```python
from build123d import *

# Parameters (mm, degrees)
BOSS_EXTRUDE1_DEPTH     = 6
CUT_EXTRUDE1_START      = 3
SKETCH2_R               = 8.25
CUT_EXTRUDE1_DEPTH      = 3
CUT_EXTRUDE2_REACH      = 14
SKETCH3_R               = 1.75
SKETCH4_R               = 3
CUT_EXTRUDE3_DEPTH      = 1
CUT_EXTRUDE3_DEPTH_BACK = 3


with BuildPart() as part:
    # Sketch1 → Boss-Extrude1 (new body, symmetric)
    with BuildSketch(Plane(origin=(0, 0, 0), x_dir=(1, 0, 0), z_dir=(0, 1, 0))):
        with BuildLine():
            Line((-6.25, 0), (-18.75, 0))
            Line((-18.75, 0), (-18.75, 12))
            Line((-18.75, 12), (18.75, 12))
            Line((18.75, 12), (18.75, 0))
            Line((18.75, 0), (6.25, 0))
            ThreePointArc((6.25, 0), (0, 6.25), (-6.25, 0))
        make_face()
    extrude(amount=BOSS_EXTRUDE1_DEPTH, both=True)

    # Sketch2 → Cut-Extrude1 (cut)
    with BuildSketch(Plane(origin=(0, 0, 0), x_dir=(1, 0, 0), z_dir=(0, 1, 0)).offset(CUT_EXTRUDE1_START)):
        Circle(SKETCH2_R)
    cut_extrude1 = extrude(amount=CUT_EXTRUDE1_DEPTH, mode=Mode.SUBTRACT)

    # Mirror1: Cut-Extrude1 across plane
    add(cut_extrude1.mirror(Plane.ZX), mode=Mode.SUBTRACT)

    # Sketch3 → Cut-Extrude2 (cut, up to next)
    with BuildSketch(Plane.XY, mode=Mode.PRIVATE) as cut_extrude2_sk1:
        with Locations((-11.25, 0)):
            Circle(SKETCH3_R)
    cut_extrude2_tool1 = extrude(cut_extrude2_sk1.sketch, amount=-CUT_EXTRUDE2_REACH, mode=Mode.PRIVATE) & part.part
    add(cut_extrude2_tool1.solids().sort_by_distance((-11.25, 0, 0))[0], mode=Mode.SUBTRACT)
    # Sketch3 → Cut-Extrude2 (cut, up to next)
    with BuildSketch(Plane.XY, mode=Mode.PRIVATE) as cut_extrude2_sk2:
        with Locations((11.25, 0)):
            Circle(SKETCH3_R)
    cut_extrude2_tool2 = extrude(cut_extrude2_sk2.sketch, amount=-CUT_EXTRUDE2_REACH, mode=Mode.PRIVATE) & part.part
    add(cut_extrude2_tool2.solids().sort_by_distance((11.25, 0, 0))[0], mode=Mode.SUBTRACT)

    # Sketch4 → Cut-Extrude3 (cut, two sides)
    with BuildSketch(Plane(origin=(0, 0, -12), x_dir=(-1, 0, 0), z_dir=(0, 0, -1))) as cut_extrude3_sk:
        with Locations((11.25, 0)):
            Circle(SKETCH4_R)
        with Locations((-11.25, 0)):
            Circle(SKETCH4_R)
    extrude(amount=CUT_EXTRUDE3_DEPTH, mode=Mode.SUBTRACT)
    extrude(cut_extrude3_sk.sketch, amount=-CUT_EXTRUDE3_DEPTH_BACK, mode=Mode.SUBTRACT)


solid = part.part
```
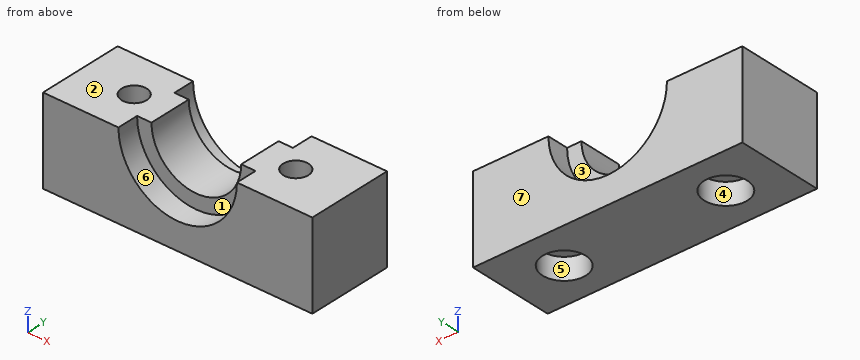
CAD build for the part. Positions are in the model's coordinates, mm. Face numbers are marked on the shaded views. A direction names the side the tool comes from. Round coordinates to 2 decimals unless told otherwise and drop trailing zeros. Loops run counter-clockwise (first coordinate to the right, second up) from the corner with the lowest first, then second, coordinate; pieces in that order, holes last. Notation, with made-up numbers: (-30.5, -38.75) - (-23.5, -38.75) arc R19 cw to (-23.5, -33.75) - close; hole circle Ø4 at (57, 33). An arc over 180 degrees is marked (long way). Return JSON: item names as keys, results as strings. Group by question number.
Q1. Drill centre lines: line 1 along Y through (x, z) = (-11.25, -6.75); line 2 along Y through (x, z) = (-11.25, -10.7); line 3 along X through (y, z) = (0.75, -3.25). Where is each one in solid material? Low to high. Write a range as [from, to].
Q2. Band-saw the part on A-A on z = -3. Give the cut face in (x, y).
Q3. Two-plate mould, pull along Y, no slides. Class the marked faces 1, 2, 3 and 4: +Y half, -Y half, draft (parallel to the pull), parting line (faces both ways), or undercut.
Q4. Flat gauge pins, fed straight in: pin 1 Ø5 at (x, y) = (-12.5, 1) entering from -Z; pin 2 Ø5.5 at (x, y) = (-11.25, 0) entering from -Z; pin 3 Ø5 at (x, y) = (-2, 0.5) entering from +Z; pin 4 Ø2.5 at (x, z) = (-3.5, -5.5) entering from +Y. Where does each tip first touch, or does it go through?
Q5. Band-saw the part on D-D on x = -4. Give the cut face in (y, z), plus the area to 3 significant figures.
Q6. Band-saw the part on C-C on y = 3.5. Give the cut face in (x, z).
Q7. Tool access for the marked faces 5, 6 and 7: list every direction of +Z, -Z, +X, -X, +Y, -Y with a clear straight run to the whole face (end or side of a thin tool).
Q8. Band-saw the part on B-B on x = -11.25. Give the cut face in (y, z).
Solutions:
{
 "1": {"line 1": "y = [-6, -1.75], [1.75, 6]", "line 2": "y = [-6, -3], [3, 6]", "line 3": "x = [-18.75, -12.83], [-9.67, -5.34], [5.34, 9.67], [12.83, 18.75]"},
 "2": {"outline": "(-18.75, -6) - (-7.69, -6) - (-7.69, -3) - (-5.48, -3) - (-5.48, 3) - (-7.69, 3) - (-7.69, 6) - (-18.75, 6) - close; (5.48, -3) - (7.69, -3) - (7.69, -6) - (18.75, -6) - (18.75, 6) - (7.69, 6) - (7.69, 3) - (5.48, 3) - close; hole circle Ø3.5 at (-11.25, 0); hole circle Ø3.5 at (11.25, 0)"},
 "3": {"face 1": "-Y half", "face 2": "draft", "face 3": "+Y half", "face 4": "undercut"},
 "4": {"pin 1": "stops at z = -12", "pin 2": "stops at z = -9", "pin 3": "stops at z = -4.34", "pin 4": "stops at y = 3"},
 "5": {"outline": "(-6, -12) - (6, -12) - (6, -7.22) - (3, -7.22) - (3, -4.8) - (-3, -4.8) - (-3, -7.22) - (-6, -7.22) - close", "area": "71.9 mm^2"},
 "6": {"outline": "(-18.75, -12) - (18.75, -12) - (18.75, 0) - (8.25, 0) arc R8.25 cw to (-8.25, 0) - (-18.75, 0) - close"},
 "7": {"face 5": "-Z", "face 6": "+Z, -Y", "face 7": "+Z, -Z, +X, -X, +Y"},
 "8": {"outline": "(-6, -12) - (-3, -12) - (-3, -9) - (-1.75, -9) - (-1.75, 0) - (-6, 0) - close; (1.75, -9) - (3, -9) - (3, -12) - (6, -12) - (6, 0) - (1.75, 0) - close"}
}
